Source: CAD feature listing. Evaluate the final solid. Frame: model axes, mm. Give positions to 0.01 mm unless a question says otherwise; leave off trailing zeros. Loops run counter-clockwise (first coordinate to the right, second up) from the corner with the lowest first, then second, coordinate; pieces in that order, holes last. Notation, with made-up numbers: M -8,-24 L 20,-24 A21 cw 20,1 Z; hole C 4,44.25 d10. An arc over 180 degrees is marked long. Answer in a Markdown table with one row per item.
```python
from build123d import *

# Parameters (mm, degrees)
SALIENTE_EXTRUIR1_DEPTH   = 2.4
SALIENTE_EXTRUIR1_2_DEPTH = 2.4
SALIENTE_EXTRUIR2_DEPTH   = 1


with BuildPart() as part:
    # Croquis1 → Saliente-Extruir1 (new body)
    with BuildSketch(Plane.XY):
        with BuildLine():
            Line((-24.903989872, 3.946781248), (-25.3, 4))
            ThreePointArc((-25.3, 4), (-26.8, 2.5), (-25.3, 1))
            ThreePointArc((-25.3, 1), (-24.239339828, 1.439339828), (-23.8, 2.5))
            ThreePointArc((-23.8, 2.5), (-24.1075204, 3.409940879), (-24.903989872, 3.946781248))
        make_face()
    extrude(amount=SALIENTE_EXTRUIR1_DEPTH)



with BuildPart() as body_2:
    # Croquis1 → Saliente-Extruir1 2 (new body)
    with BuildSketch(Plane.XY):
        with BuildLine():
            ThreePointArc((0.6, 0), (0.424264069, 0.424264069), (0, 0.6))
            ThreePointArc((0, 0.6), (-0.598803756, 0.037869012), (-0.075587022, -0.595219793))
            Line((-0.075587022, -0.595219793), (0, -0.6))
            ThreePointArc((0, -0.6), (0.424264069, -0.424264069), (0.6, 0))
        make_face()
    extrude(amount=SALIENTE_EXTRUIR1_2_DEPTH)


with BuildPart() as part_1:
    add(part.part)

    add(body_2.part)  # Saliente-Extruir2 merges body 2
    # Croquis1_3 → Saliente-Extruir2 (add)
    with BuildSketch(Plane.XY):
        with BuildLine():
            Line((0, 0.6), (-24.903989872, 3.946781248))
            ThreePointArc((-24.903989872, 3.946781248), (-24.1075204, 3.409940879), (-23.8, 2.5))
            ThreePointArc((-23.8, 2.5), (-24.239339828, 1.439339828), (-25.3, 1))
            Line((-25.3, 1), (-0.075587022, -0.595219793))
            ThreePointArc((-0.075587022, -0.595219793), (-0.598803756, 0.037869012), (0, 0.6))
        make_face()
    extrude(amount=SALIENTE_EXTRUIR2_DEPTH)


solid = part_1.part
```
1) Section D-D, the plane x = -15.5. Return loops of the section in (y, z), then the cut area to 3 significant figures.
Reply:
| item | result |
|---|---|
| outline | M 0.38,0 L 2.68,0 L 2.68,1 L 0.38,1 Z |
| area | 2.30 mm² |
2) Material intervals for L1, parallel to X at y = 2.4, z = 1.1; L2, parallel to Z at x = -19.75, y = 2.9; L3, parallel to Y at x = -8.5, z = 0.75, sorted ascending.
Reply:
| item | result |
|---|---|
| L1 | x = -26.8 to -23.8 |
| L2 | z = 0 to 1 |
| L3 | y = -0.06 to 1.74 |
3) Section B-B, the plane z = 0.4. Return loops of the section in (x, y).
Reply:
| item | result |
|---|---|
| outline | M -25.3,1 L 0,-0.6 A0.6 ccw 0,0.6 L -25.3,4 A1.5 ccw Z |
4) Section C-C, the plane y = 1.5. Return loops of the section in (x, z).
Reply:
| item | result |
|---|---|
| outline | M -26.42,0 L -6.7,0 L -6.7,1 L -24.18,1 L -24.18,2.4 L -26.42,2.4 Z |
5) Pin query (flat end, axial travel): pin 1 Ø1 at (x, z) = (-5, 1) entering from +Y; pin 2 Ø1 at (x, y) = (-22.5, 3) entering from +Z. Return the tip coordinate at first contact, or that it passes through.
Reply:
| item | result |
|---|---|
| pin 1 | stops at y = 1.34 |
| pin 2 | stops at z = 1 |
6) Section A-A, the plane z = 2. Return loops of the section in (x, y).
Reply:
| item | result |
|---|---|
| outline | M -25.3,4 A1.5 ccw long -24.9,3.95 Z; M -0.08,-0.6 L 0,-0.6 A0.6 ccw long Z |
